Design review of the part built by this model. Coordinates are the model's own, in mm. A direction names the side the tool comes from. Round coordinates to 2 decimals unless told otherwise and drop trailing zeros. Loops run counter-clockwise (first coordinate to the right, second up) from the corner with the lowest first, then second, coordinate; pieces in that order, holes last. Notation, with made-up numbers: M 34,-31.75 L 50,-31.75 A15 cw 50,-15.75 Z; hole C 64.25,62.25 d4. An arc over 180 degrees is marked long. One line per item, written item: value. Start each with the question number.
Item 1: We need section A-A (z = -4.5). Write out the cut boundary in (x, y).
Item 2: Mouldability with a two-part tool opening along Z and no side actions: class faces 4 (the flat face through (-166.141, -133, 40)), 5 (the flat face through (-51, -137, 35)) as released by +Z, released by -Z, zero draft, split by the parting line, or undercut.
Item 3: We need section D-D (y = -94). Write out the cut boundary in (x, z), then the cut area to 3 significant figures.
Item 4: Clearance check with flat-ended pins moving along their axes: pin 1 (3.5 mm diameter, centred on y = -138.5, z = 20.5, fed in from -X); pin 2 (11 mm diameter, centred on y = -119, z = -3.5, fed in from +X); pin 3 (2 mm diameter, centred on x = -84.5, y = -136, fed in from -Z). State where each tip first meets the part, or that it passes through.
Item 5: We need section B-B (y = -128). Write out the cut boundary in (x, z), then the cut area to 3 significant figures.
Item 6: We need section C-C (x = -33.5). Write out the cut boundary in (y, z), then the cut area to 3 significant figures.
Item 7: For line 1 along X through (y, z) = (-127, 39.5); line 2 along X through (y, z) = (-122, 41.5); line 3 along Z through (x, y) = (-14.5, -123), list the stretches that pass through material, from the lowest coordinate up.
Item 8: For faces 1 (the flat face through (-46.071, -137.013, 22.675)), 2 (the flat face through (-121.141, -107, 4)), 3 (the flat face through (-44, -133.464, -5)), list the 3-axis set-ups (+Z, -Z, +X, -X, +Y, -Y) from which the entire face can be reached by the end or side of a thin tool; tool diameter is ignored.
from build123d import *

# Parameters (mm, degrees)
ESQUISSE2_W             = 15
ESQUISSE2_H             = 33
ESQUISSE2_R             = 1
ESQUISSE2_W_2           = 70
ESQUISSE2_H_2           = 7
BOSS_EXTRU_1_DEPTH      = 10
ESQUISSE3_W             = 150
ESQUISSE3_H             = 7
BOSS_EXTRU_2_DEPTH      = 40
ESQUISSE4_W             = 40
ESQUISSE4_H             = 20
ESQUISSE4_R             = 1
ESQUISSE4_W_2           = 5
ESQUISSE4_H_2           = 15
BOSS_EXTRU_3_DEPTH      = 20
ENL_V_MAT_EXTRU_1_DEPTH = 181.562942337
ESQUISSE6_W             = 40
ESQUISSE6_H             = 20
ENL_V_MAT_EXTRU_2_DEPTH = 10
CONG_1_R                = 10
BOSS_EXTRU_4_DEPTH      = 10


with BuildPart() as part:
    # Esquisse2 → Boss.-Extru.1 (new body)
    # profile 1 of 5: a face of its own
    with BuildSketch(Plane.XY):
        Polygon((-121.141434162, -90.464178298), (-161.141434162, -90.464178298), (-161.141434162, -140.464178298), (-121.141434162, -140.464178298), (-121.141434162, -133.464178298), (-136.141434162, -133.464178298), (-136.141434162, -100.464178298), (-121.141434162, -100.464178298), align=None)
    # profile 2 of 5: a face of its own
    with BuildSketch(Plane.XY):
        with Locations((-128.641434162, -116.964178298)):
            Rectangle(ESQUISSE2_W, ESQUISSE2_H)
        with Locations((-126.141434162, -123.464178298)):
            Circle(ESQUISSE2_R, mode=Mode.SUBTRACT)
        with Locations((-126.141434162, -110.464178298)):
            Circle(ESQUISSE2_R, mode=Mode.SUBTRACT)
    # profile 3 of 5: a face of its own
    with BuildSketch(Plane.XY):
        with Locations((-86.141434162, -136.964178298)):
            Rectangle(ESQUISSE2_W_2, ESQUISSE2_H_2)
    # profile 4 of 5: a face of its own
    with BuildSketch(Plane.XY):
        with Locations((-43.641434162, -116.964178298)):
            Rectangle(ESQUISSE2_W, ESQUISSE2_H)
        with Locations((-46.141434162, -123.464178298)):
            Circle(ESQUISSE2_R, mode=Mode.SUBTRACT)
        with Locations((-46.141434162, -110.464178298)):
            Circle(ESQUISSE2_R, mode=Mode.SUBTRACT)
    # profile 5 of 5: a face of its own
    with BuildSketch(Plane.XY):
        Polygon((-51.141434162, -133.464178298), (-51.141434162, -140.464178298), (-11.141434162, -140.464178298), (-11.141434162, -90.464178298), (-51.141434162, -90.464178298), (-51.141434162, -100.464178298), (-36.141434162, -100.464178298), (-36.141434162, -133.464178298), align=None)
    extrude(amount=BOSS_EXTRU_1_DEPTH)

    # Esquisse3 → Boss.-Extru.2 (add)
    with BuildSketch(Plane.XY.offset(10)):
        with Locations((-86.141434162, -136.964178298)):
            Rectangle(ESQUISSE3_W, ESQUISSE3_H)
    extrude(amount=BOSS_EXTRU_2_DEPTH)

    # Esquisse4 → Boss.-Extru.3 (add)
    # profile 1 of 4: a face of its own
    with BuildSketch(Plane.XY.offset(50)):
        with Locations((-141.141434162, -123.464178298)):
            Rectangle(ESQUISSE4_W, ESQUISSE4_H)
        with Locations((-151.141434162, -123.464178298)):
            Circle(ESQUISSE4_R, mode=Mode.SUBTRACT)
        with Locations((-131.141434162, -123.464178298)):
            Circle(ESQUISSE4_R, mode=Mode.SUBTRACT)
    # profile 2 of 4: a face of its own
    with BuildSketch(Plane.XY.offset(50)):
        with Locations((-31.141434162, -123.464178298)):
            Rectangle(ESQUISSE4_W, ESQUISSE4_H)
        with Locations((-41.141434162, -123.464178298)):
            Circle(ESQUISSE4_R, mode=Mode.SUBTRACT)
        with Locations((-21.141434162, -123.464178298)):
            Circle(ESQUISSE4_R, mode=Mode.SUBTRACT)
    # profile 3 of 4: a face of its own
    with BuildSketch(Plane.XY.offset(50)):
        with Locations((-163.641434162, -132.964178298)):
            Rectangle(ESQUISSE4_W_2, ESQUISSE4_H_2)
    # profile 4 of 4: a face of its own
    with BuildSketch(Plane.XY.offset(50)):
        with Locations((-8.641434162, -132.964178298)):
            Rectangle(ESQUISSE4_W_2, ESQUISSE4_H_2)
    extrude(amount=-BOSS_EXTRU_3_DEPTH)

    # Esquisse5 → Enlèv. mat.-Extru.1 (cut, through all)
    with BuildSketch(Plane.XZ.offset(140.464178298)):
        Polygon((-151.141434162, 35), (-151.141434162, 10), (-141.141434162, 10), align=None)
        Polygon((-146.141434162, 35), (-136.141434162, 10), (-136.141434162, 35), align=None)
        Polygon((-131.141434162, 35), (-131.141434162, 10), (-121.141434162, 10), align=None)
        Polygon((-126.141434162, 35), (-116.141434162, 10), (-116.141434162, 35), align=None)
        Polygon((-101.141434162, 35), (-91.141434162, 10), (-81.141434162, 10), (-71.141434162, 35), align=None)
        Polygon((-111.141434162, 35), (-111.141434162, 10), (-101.141434162, 10), align=None)
        Polygon((-71.141434162, 10), (-61.141434162, 10), (-61.141434162, 35), align=None)
        Polygon((-46.141434162, 35), (-56.141434162, 35), (-56.141434162, 10), align=None)
        Polygon((-41.141434162, 35), (-51.141434162, 10), (-41.141434162, 10), align=None)
        Polygon((-21.141434162, 35), (-21.141434162, 10), (-31.141434162, 35), align=None)
        Polygon((-36.141434162, 35), (-36.141434162, 10), (-26.141434162, 10), align=None)
    extrude(amount=-ENL_V_MAT_EXTRU_1_DEPTH, mode=Mode.SUBTRACT)

    # Esquisse6 → Enlèv. mat.-Extru.2 (cut)
    with BuildSketch(Plane(origin=(0, 0, 30), x_dir=(-1, 0, 0), z_dir=(0, 0, -1))):
        with Locations((31.141434162, -123.464178298)):
            Rectangle(ESQUISSE6_W, ESQUISSE6_H)
        with Locations((141.141434162, -123.464178298)):
            Rectangle(ESQUISSE6_W, ESQUISSE6_H)
    extrude(amount=-ENL_V_MAT_EXTRU_2_DEPTH, mode=Mode.SUBTRACT)

    # Congé1
    # the kernel refuses this fillet: 10 mm, written as the material it takes off along each edge
    with BuildSketch(Plane(origin=(18.858565838, -140.464178298, 50), x_dir=(0, 1, 0), z_dir=(-1, 0, 0))) as cong_1_piece_1:
        with BuildLine():
            CenterArc((CONG_1_R, CONG_1_R), CONG_1_R, 180, 90)
            Line((0, CONG_1_R), (0, 0))
            Line((0, 0), (CONG_1_R, 0))
        make_face()
    extrude(amount=210, mode=Mode.SUBTRACT)

    # Esquisse7 → Boss.-Extru.4 (add)
    with BuildSketch(Plane(origin=(0, 0, 0), x_dir=(-1, 0, 0), z_dir=(0, 0, -1))):
        Polygon((51.141434162, -100.464178298), (51.141434162, -90.464178298), (21.141434162, -90.464178298), (21.141434162, -140.464178298), (51.141434162, -140.464178298), (51.141434162, -133.464178298), (36.141434162, -133.464178298), (36.141434162, -100.464178298), align=None)
        Polygon((121.141434162, -133.464178298), (121.141434162, -140.464178298), (151.141434162, -140.464178298), (151.141434162, -90.464178298), (121.141434162, -90.464178298), (121.141434162, -100.464178298), (136.141434162, -100.464178298), (136.141434162, -133.464178298), align=None)
    extrude(amount=BOSS_EXTRU_4_DEPTH)


solid = part.part
A:
1. outline: M -151.14,-140.46 L -121.14,-140.46 L -121.14,-133.46 L -136.14,-133.46 L -136.14,-100.46 L -121.14,-100.46 L -121.14,-90.46 L -151.14,-90.46 Z; M -51.14,-140.46 L -21.14,-140.46 L -21.14,-90.46 L -51.14,-90.46 L -51.14,-100.46 L -36.14,-100.46 L -36.14,-133.46 L -51.14,-133.46 Z
2. face 4: zero draft
2. face 5: undercut
3. outline: M -161.14,0 L -151.14,0 L -151.14,-10 L -121.14,-10 L -121.14,10 L -161.14,10 Z; M -51.14,-10 L -21.14,-10 L -21.14,0 L -11.14,0 L -11.14,10 L -51.14,10 Z
3. area: 1,400 mm2
4. pin 1: x = -161.14
4. pin 2: x = -11.14
4. pin 3: z = 0
5. outline: M -166.14,30 L -161.14,30 L -161.14,40 L -121.14,40 L -121.14,50 L -166.14,50 Z; M -161.14,0 L -151.14,0 L -151.14,-10 L -136.14,-10 L -136.14,0 L -121.14,0 L -121.14,10 L -161.14,10 Z; M -51.14,0 L -36.14,0 L -36.14,-10 L -21.14,-10 L -21.14,0 L -11.14,0 L -11.14,10 L -51.14,10 Z; M -51.14,40 L -11.14,40 L -11.14,30 L -6.14,30 L -6.14,50 L -51.14,50 Z
5. area: 2,100 mm2
6. outline: M -140.46,-10 L -90.46,-10 L -90.46,10 L -140.46,10 Z; M -140.46,28.4 L -133.46,28.4 L -133.46,40 L -113.46,40 L -113.46,50 L -130.46,50 A10 ccw -140.46,40 Z
6. area: 1,330 mm2
7. line 1: -166.14 to -161.14, -11.14 to -6.14
7. line 2: -161.14 to -121.14, -51.14 to -11.14
7. line 3: 0 to 10, 40 to 50
8. face 1: +Y, -Y
8. face 2: +Z, -Z, +Y
8. face 3: -Z
